```python
from build123d import *

# Parameters (mm, degrees)
SKETCH1_W               = 25.4
SKETCH1_H               = 25.4
SKETCH1_W_2             = 19.05
SKETCH1_H_2             = 19.05
EXTRUDE1_DEPTH          = 25.4
SKETCH3_R               = 4.0005
SKETCH3_R_2             = 1.1938
CUT_EXTRUDE1_DEPTH      = 25.6126
CUT_EXTRUDE1_DEPTH_BACK = 25.4
SKETCH2_R               = 1.1938
SKETCH2_R_2             = 4.0005
CUT_EXTRUDE2_DEPTH      = 25.6126
CUT_EXTRUDE2_DEPTH_BACK = 25.4


with BuildPart() as part:
    # Sketch1 → Extrude1 (new body)
    with BuildSketch(Plane(origin=(0, 0, 0), x_dir=(0, 0, -1), z_dir=(1, 0, 0))):
        with Locations((-11.9126, 11.9126)):
            Rectangle(SKETCH1_W, SKETCH1_H)
        with Locations((-11.9126, 11.9126)):
            Rectangle(SKETCH1_W_2, SKETCH1_H_2, mode=Mode.SUBTRACT)
    extrude(amount=EXTRUDE1_DEPTH)

    # Sketch3 → Cut-Extrude1 (cut, two sides)
    with BuildSketch(Plane(origin=(0, 0, 0), x_dir=(1, 0, 0), z_dir=(0, 1, 0))) as cut_extrude1_sk:
        with Locations(Location((12.7, -11.9126, 0), (0, 0, 90))):  # turned: the seam where the file's is
            Circle(SKETCH3_R)
        with Locations(Location((4.3688, -11.9126, 0), (0, 0, 90))):  # turned: the seam where the file's is
            Circle(SKETCH3_R_2)
        with Locations(Location((21.0312, -11.9126, 0), (0, 0, 90))):  # turned: the seam where the file's is
            Circle(SKETCH3_R_2)
    extrude(amount=CUT_EXTRUDE1_DEPTH, mode=Mode.SUBTRACT)
    extrude(cut_extrude1_sk.sketch, amount=-CUT_EXTRUDE1_DEPTH_BACK, mode=Mode.SUBTRACT)

    # Sketch2 → Cut-Extrude2 (cut, two sides)
    with BuildSketch(Plane.XY) as cut_extrude2_sk:
        with Locations((4.3688, 11.9126)):
            Circle(SKETCH2_R)
        with Locations((21.0312, 11.9126)):
            Circle(SKETCH2_R)
        with Locations((12.7, 11.9126)):
            Circle(SKETCH2_R_2)
    extrude(amount=CUT_EXTRUDE2_DEPTH, mode=Mode.SUBTRACT)
    extrude(cut_extrude2_sk.sketch, amount=-CUT_EXTRUDE2_DEPTH_BACK, mode=Mode.SUBTRACT)


solid = part.part
```
Geometry check sheet. Reference: the model listing, model coordinates, mm. A direction names the side the tool comes from. Coordinates: 2 decimals unless noted, no trailing zeros. Loops run counter-clockwise (first coordinate to the right, second up) from the corner with the lowest first, then second, coordinate; pieces in that order, holes last. Notation, with made-up numbers: (71, -27) -> (101, -27) arc R29 ccw to (101, 3) -> close; hole circle Ø11 at (83.5, 74.25). An arc over 180 degrees is marked (long way). Put each result on its own line as item: value.
1) Cross-section at D-D on x = 12.7. Record the boundary of the cut face in (y, z).
Result set:
outline: (-0.79, -0.79) -> (7.91, -0.79) -> (7.91, 2.39) -> (2.39, 2.39) -> (2.39, 7.91) -> (-0.79, 7.91) -> close; (-0.79, 15.91) -> (2.39, 15.91) -> (2.39, 21.44) -> (7.91, 21.44) -> (7.91, 24.61) -> (-0.79, 24.61) -> close; (15.91, -0.79) -> (24.61, -0.79) -> (24.61, 7.91) -> (21.44, 7.91) -> (21.44, 2.39) -> (15.91, 2.39) -> close; (15.91, 21.44) -> (21.44, 21.44) -> (21.44, 15.91) -> (24.61, 15.91) -> (24.61, 24.61) -> (15.91, 24.61) -> close
2) Gauge pin test, flat ends, axial feed: pin 1 Ø5 at (x, y) = (12.7, 11.91) entering from -Z; pin 2 Ø13 at (x, z) = (12.7, 11.91) entering from +Y. Record the tip position at first contact, or that the pin passes through.
Result set:
pin 1: passes through
pin 2: stops at y = 24.61
3) Cross-section at B-B on x = 18. Record the boundary of the cut face in (y, z).
Result set:
outline: (-0.79, -0.79) -> (24.61, -0.79) -> (24.61, 24.61) -> (-0.79, 24.61) -> close; hole (2.39, 2.39) -> (21.44, 2.39) -> (21.44, 21.44) -> (2.39, 21.44) -> close
4) Thickness scan on line 1 (Y direction, x = 3.5, z = 13); line 2 (X direction, y = 13.5, z = 1). Record the ranges inside material, lowest first.
Result set:
line 1: y = -0.79 to 2.39, 21.44 to 24.61
line 2: x = 0 to 9.03, 16.37 to 25.4
5) Cross-section at A-A on z = 7.25. Record the boundary of the cut face in (x, y), plus the area to 3 significant figures.
Result set:
outline: (0, -0.79) -> (25.4, -0.79) -> (25.4, 2.39) -> (0, 2.39) -> close; (0, 21.44) -> (25.4, 21.44) -> (25.4, 24.61) -> (0, 24.61) -> close
area: 161 mm^2
6) Release check for a two-part mould opening along Y. For faces 3 (the flat face through (9.7, 24.613, 14.9)), 4 (the cylindrical face through (12.18, 15.88, 23)), 5 (the flat face through (9.7, -0.787, 14.9)) record: released by +Y, released by -Y, zero draft, split by the parting line, or undercut.
Result set:
face 3: released by +Y
face 4: undercut
face 5: released by -Y
7) Tool access check on faces 1 (the flat face through (12.5, 21.438, 16.3)), 2 (the cylindrical face through (15.13, 23, 15.09)). Record the directions out of +Z, -Z, +X, -X, +Y, -Y that give a thin tool (end or side, any length) a straight path to the whole face; none if there is none.
Result set:
face 1: +X, -X
face 2: +Y, -Y
